Can you work these out from the model? Positions are in its coordinate system, mm. Give positions to 0.01 mm unless a question says otherwise; leave off trailing zeros. Order: outer loops, then holes, each group sorted by start corner. A loop starts at its lowest first (then second) coordinate and runs counter-clockwise, first axis right, second up. Notation, with made-up numbers: (52, -39.5) - (74, -39.5) arc R18 cw to (74, -25.5) - close; hole circle Ø5 at (-20.75, -13). An arc over 180 degrees is marked (long way). Use one line per item in the form item = value. Start each with the question number.
1) Suppose I cut it at B-B, the plane x = -30.5. Write out the boundary of the cut face in (y, z).
2) Please list where these lines run through material, in increasing order: probe 1 along Y at (x, z) = (-28.5, 3); probe 2 along X at (y, z) = (-11.5, 0); probe 3 along X at (y, z) = (9, 4.5).
3) For pin 1 (1 mm diameter, centred on x = -29, z = -8.5, fed in from -Y); pin 2 (4 mm diameter, centred on y = 6, z = -8, fed in from +X); pin 3 (12 mm diameter, centred on y = 15, z = -35.5, fed in from -X), each with a flat end and sliding along its axis, tell me the tip position at first contact or that it passes through.
4) Suppose I cut it at A-A, the plane y = -5.5. Write out the boundary of the cut face in (x, z) (3 decimals).
```python
from build123d import *

# Parameters (mm, degrees)
BOSS_EXTRUDE1_DEPTH    = 1.6
BACK_MOUNTING_HOLES_R  = 1.7
CUT_EXTRUDE1_DEPTH     = 11.983113317
FRONT_MOUNTING_HOLES_R = 1.7
CUT_EXTRUDE2_DEPTH     = 11.983113317


with BuildPart() as part:
    # Sketch1 → Boss-Extrude1 (new body)
    with BuildSketch(Plane(origin=(-29.019700562, 0, 4.594785922), x_dir=(-0.156385222, 0, -0.987696139), z_dir=(0.987696139, 0, -0.156385222))):
        Polygon((-6.520440675, 24.056053189), (54.226987254, 25), (54.226987254, -25), (-6.520440675, -24.056053189), align=None)
    extrude(amount=BOSS_EXTRUDE1_DEPTH)

    # Back Mounting Holes → Cut-Extrude1 (cut, through all)
    with BuildSketch(Plane(origin=(-29.019700562, 0, 4.594785922), x_dir=(0.156385222, 0, 0.987696139), z_dir=(-0.987696139, 0, 0.156385222))):
        with Locations((1.520440675, -11)):
            Circle(BACK_MOUNTING_HOLES_R)
        with Locations((1.520440675, 11)):
            Circle(BACK_MOUNTING_HOLES_R)
    extrude(amount=-CUT_EXTRUDE1_DEPTH, mode=Mode.SUBTRACT)

    # Front Mounting Holes → Cut-Extrude2 (cut, through all)
    with BuildSketch(Plane(origin=(-29.019700562, 0, 4.594785922), x_dir=(0.156385222, 0, 0.987696139), z_dir=(-0.987696139, 0, 0.156385222))):
        with Locations((-49.726987254, 15)):
            Circle(FRONT_MOUNTING_HOLES_R)
        with Locations((-49.726987254, -15)):
            Circle(FRONT_MOUNTING_HOLES_R)
    extrude(amount=-CUT_EXTRUDE2_DEPTH, mode=Mode.SUBTRACT)


solid = part.part
```
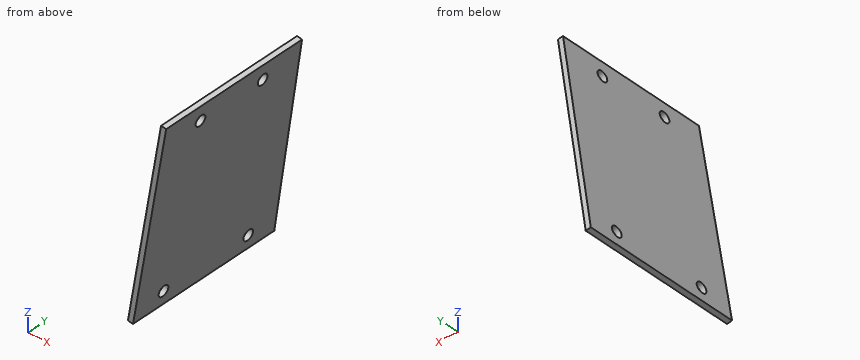
Result sheet:
q1.outline = (-24.46, -14.99) - (24.46, -14.99) - (24.3, -4.75) - (-24.3, -4.75) - close
q2.probe_1 = -24.18 to 24.18
q2.probe_2 = -29.75 to -28.13
q2.probe_3 = -29.03 to -27.41
q3.pin_1 = -24.36
q3.pin_2 = -29.08
q3.pin_3 = -36.32
q4.outline = (-37.5, -48.965) - (-35.92, -49.215) - (-26.42, 10.785) - (-28, 11.035) - close
